The listing builds one solid part. Answer for the finished solid, in the listing's coordinates (mm). Face numbers are marked on the shaded views. A direction names the side the tool comes from. Round coordinates to 2 decimals unless told otherwise and drop trailing zeros. Loops run counter-clockwise (first coordinate to the right, second up) from the corner with the lowest first, then second, coordinate; pieces in that order, holes last. Notation, with made-up numbers: (31, 44) - (66, 44) arc R32 cw to (66, 73) - close; hole circle Ø10 at (3.25, 23.5). An arc over 180 degrees is marked (long way). One line per item, written item: value.
```python
from build123d import *

# Parameters (mm, degrees)
F0_R     = 25
F1_DEPTH = 20
F3_R     = 25
F4_DEPTH = 10
F5_W     = 50
F5_H     = 100
F6_DEPTH = 20


with BuildPart() as f1:
    # F0 (on Front) → F1 (new body)
    with BuildSketch(Plane.XZ):
        with BuildLine():
            Line((-100, -50), (0, -50))
            ThreePointArc((0, -50), (50, 0), (0, 50))
            Line((0, 50), (-100, 50))
            Line((-100, 50), (-100, -50))
        make_face()
        Circle(F0_R, mode=Mode.SUBTRACT)
    extrude(amount=F1_DEPTH)



with BuildPart() as f4:
    # F3 (on offset) → F4 (new body)
    with BuildSketch(Plane.XZ.offset(40)):
        with BuildLine():
            Line((-100, 50), (-100, -50))
            Line((-100, -50), (0, -50))
            ThreePointArc((0, -50), (50, 0), (0, 50))
            Line((0, 50), (-100, 50))
        make_face()
        Circle(F3_R, mode=Mode.SUBTRACT)
    extrude(amount=F4_DEPTH)


with BuildPart() as f1_1:
    add(f1.part)

    add(f4.part)  # F6 merges F4
    # F5 (on face) → F6 (join, through all)
    with BuildSketch(Plane.XZ.offset(20)):
        with Locations((-75, 0)):
            Rectangle(F5_W, F5_H)
    extrude(amount=F6_DEPTH)


solid = f1_1.part
```
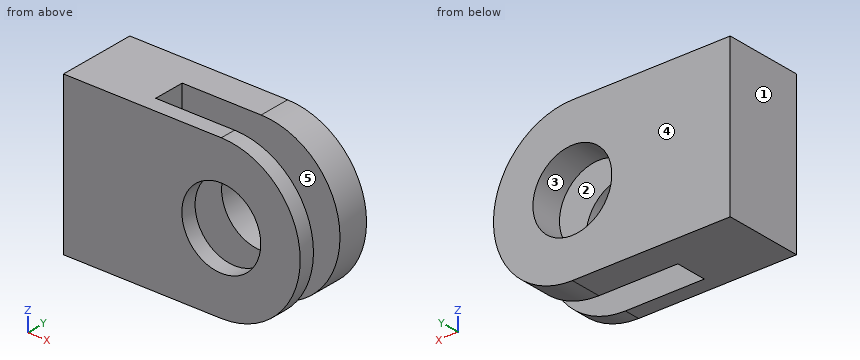
1) A cutting plane is placed at C-C on x = -7. Give the vertices of the cut face in (y, z).
Final values:
outline: (-50, -50) - (-40, -50) - (-40, -24) - (-50, -24) - close; (-50, 24) - (-40, 24) - (-40, 50) - (-50, 50) - close; (-20, -50) - (0, -50) - (0, -24) - (-20, -24) - close; (-20, 24) - (0, 24) - (0, 50) - (-20, 50) - close
2) Each of these flat-tipped pins is pushed along its axis until it touches: pin 1 Ø4 at (x, z) = (-11.5, 27.5) entering from +Y; pin 2 Ø16 at (y, z) = (-25.5, -24) entering from +X; pin 3 Ø10 at (x, z) = (-15, 7) entering from +Y; pin 4 Ø3 at (y, z) = (-36, -29) entering from +X. Where does it stop, or does it pass through?
Final values:
pin 1: y = 0
pin 2: x = 46.57
pin 3: through
pin 4: x = -50
3) Consider L1, parallel to Y at x = 22.5, z = 43; L2, parallel to X at y = -45, z = -17.5; L3, parallel to X at y = -11, z = 6. Determine where each line is inside the solid, lowest interval first.
Final values:
L1: -50 to -40, -20 to 0
L2: -100 to -17.85, 17.85 to 46.84
L3: -100 to -24.27, 24.27 to 49.64
4) A cutting plane is placed at A-A on x = -45.5. Give the vertices of the cut face in (y, z).
Final values:
outline: (-50, -50) - (-40, -50) - (-40, 50) - (-50, 50) - close; (-20, -50) - (0, -50) - (0, 50) - (-20, 50) - close
5) A cutting plane is placed at B-B on z = 0. Give the vertices of the cut face in (x, y), and give its area (3 significant figures).
Final values:
outline: (-100, -50) - (-25, -50) - (-25, -40) - (-50, -40) - (-50, -20) - (-25, -20) - (-25, 0) - (-100, 0) - close; (25, -50) - (50, -50) - (50, -40) - (25, -40) - close; (25, -20) - (50, -20) - (50, 0) - (25, 0) - close
area: 4,000 mm2
6) For a pull along X with two mould halves and no side action, classify the marked faces 1, 2 and 3 as released by +X, released by -X, zero draft, split by the parting line, or undercut.
Final values:
face 1: released by -X
face 2: zero draft
face 3: undercut
7) A cutting plane is placed at D-D on y = -14. Give the vertices of the cut face in (x, z).
Final values:
outline: (-100, -50) - (0, -50) arc R50 ccw to (0, 50) - (-100, 50) - close; hole circle Ø50 at (0, 0)
8) For the marked faces 4 and 5, determine the directions among +Z, -Z, +X, -X, +Y, -Y from which every point of the face is accessible in a straight line to the end or side of a thin tool.
Final values:
face 4: +Z, -Z, +X, -X, +Y
face 5: +Z, -Z, +X
